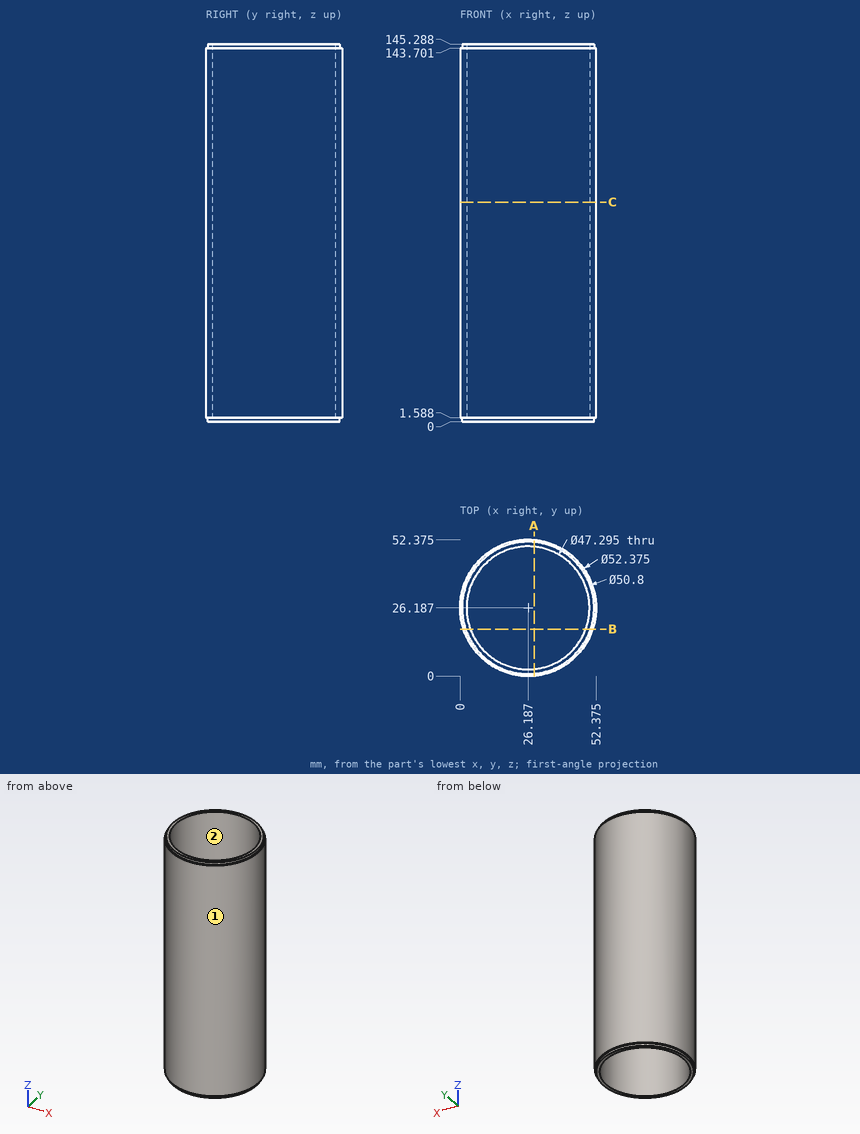
Design review of the part shown in the three views and the two pictorial views. Dimensions are in mm from the part's minimum x, y and z. Give positions to 0.01 mm unless a question says otherwise; leave off trailing zeros. Loops run counter-clockwise (first coordinate to the right, second up) from the corner with the lowest first, then second, coordinate; pieces in that order, holes last. Notation, with made-up numbers: (1.5, -31) -> (47.5, -31) arc R11 ccw to (47.5, -14) -> close; hole circle Ø4 at (17, -3). An arc over 180 degrees is marked (long way). Answer as a JSON object with one key per item and string values. Group by question number.
Q1. Take a section at A-A (x = 28.5). Write out the cut boundary in (y, z).
Q2. Take a section at C-C (z = 84.5). Write out the cut boundary in (x, y) (1 decimal).
Q3. Take a section at B-B (y = 18). Write out the cut boundary in (x, z).
Q4. Insertion check: pin 1 (3 mm diameter, centred on y = 40.5, z = 43.5, fed in from -X); pin 2 (10 mm diameter, centred on y = 14.5, z = 64, fed in from -X); pin 3 (3 mm diameter, centred on x = 40.5, z = 83, fed in from -Y). Each pin has a flat end and moves straight along its axis. Give the tip position at first contact, or say it passes through.
Q5. Draft analysis for pull direction X (two halves, no side actions). For the marked faces 1 and 2, state which applies: pulls with the +X half, pulls with the -X half, needs draft (parallel to the pull), parting line crosses it, or undercut.
Q6. Wall thickness on line 1 along Y through (x, z) = (27, 35.5) (1 decimal); line 2 along Y through (x, z) = (46, 131.5) (1 decimal); line 3 along X through (y, z) = (25, 86) (1 decimal): over which ranges is each line inside the solid? List them lowest first.
Answer below:
{
 "1": {"outline": "(0.1, 1.59) -> (0.89, 1.59) -> (0.89, 0) -> (2.65, 0) -> (2.65, 145.29) -> (0.89, 145.29) -> (0.89, 143.7) -> (0.1, 143.7) -> close; (49.72, 0) -> (51.48, 0) -> (51.48, 1.59) -> (52.27, 1.59) -> (52.27, 143.7) -> (51.48, 143.7) -> (51.48, 145.29) -> (49.72, 145.29) -> close"},
 "2": {"outline": "circle Ø52.4 at (26.2, 26.2); hole circle Ø47.3 at (26.2, 26.2)"},
 "3": {"outline": "(1.31, 1.59) -> (2.14, 1.59) -> (2.14, 0) -> (4, 0) -> (4, 145.29) -> (2.14, 145.29) -> (2.14, 143.7) -> (1.31, 143.7) -> close; (48.37, 0) -> (50.23, 0) -> (50.23, 1.59) -> (51.06, 1.59) -> (51.06, 143.7) -> (50.23, 143.7) -> (50.23, 145.29) -> (48.37, 145.29) -> close"},
 "4": {"pin 1": "stops at x = 3.35", "pin 2": "stops at x = 0.87", "pin 3": "stops at y = 3.35"},
 "5": {"face 1": "parting line crosses it", "face 2": "undercut"},
 "6": {"line 1": "y = 0 to 2.6, 49.8 to 52.4", "line 2": "y = 9.1 to 13.3, 39.1 to 43.3", "line 3": "x = 0 to 2.6, 49.8 to 52.3"}
}
